Geometry: final body of the model. Coordinates: model frame, mm. A direction names the side the tool comes from. Round coordinates to 2 decimals unless told otherwise and drop trailing zeros. Write each loop counter-clockwise with the first axis right and the second up, starting at its lowest first coordinate (ties: lowest second). Pieces come first, ordered by that corner, then holes.
Autodesk Inventor part; units mm, degrees
ref_plane "YZ Plane" through (0, 0, 0) normal (1, 0, 0) x (0, 1, 0)
ref_plane "XZ Plane" through (0, 0, 0) normal (0, 1, 0) x (-1, 0, 0)
ref_plane "XY Plane" through (0, 0, 0) normal (0, 0, 1) x (1, 0, 0)
sketch "Эскиз1" plane through (0, 0, 0) normal (0, 1, 0) x (-1, 0, 0)
  arc A0 (-11.2808, -5.3845) -> (-11.2808, 5.3845) centre (0, 0) ccw
  arc A1 (-6.7685, -3.2307) -> (-6.7685, 3.2307) centre (0, 0) ccw
  line L0 (-6.7685, -3.2307) -> (-11.2808, -5.3845)
  line L1 (-6.7685, 3.2307) -> (-11.2808, 5.3845)
  dimension "d0" = 25
  dimension "d1" = 15
extrude "Выдавливание1" add sketch "Эскиз1" along normal blind 8
sketch "Эскиз2" plane through (0, 8, 0) normal (0, 1, 0) x (1, 0, 0)
  line L0 (5.4983, 5.1008) -> (9.1638, 8.5014)
  arc A0 (11.2808, 5.3845) -> (11.2808, -5.3845) centre (0, 0) ccw
  arc A1 (11.2808, 5.3845) -> (11.2808, -5.3845) centre (0, 0) ccw
  line L1 (11.2808, -5.3845) -> (6.7685, -3.2307)
  arc A2 (6.7685, 3.2307) -> (6.7685, -3.2307) centre (0, 0) ccw
  line L2 (6.7685, 3.2307) -> (11.2808, 5.3845)
  arc A3 (6.7685, 3.2307) -> (6.7685, -3.2307) centre (0, 0) ccw
  line L3 (5.4983, -5.1008) -> (9.1638, -8.5014)
  point P0 (11.2808, -5.3845)
extrude "Выдавливание2" add sketch "Эскиз2" along normal blind 2 contours L0 A0 L2 A2 | A2 L1 A0 L3
sketch "Эскиз3" plane through (0, 8, 0) normal (0, 1, 0) x (1, 0, 0)
  arc A0 (2.2493, 8.197) -> (-2.2493, 8.197) centre (0, 0) ccw
  arc A1 (3.1548, 11.0588) -> (-3.1548, 11.0588) centre (0, 0) ccw
  line L0 (3.4451, 8.7967) -> (3.8116, 9.7325)
  arc A2 (9.1638, 8.5014) -> (9.1638, -8.5014) centre (0, 0) ccw
  arc A3 (5.4983, 5.1008) -> (5.4983, -5.1008) centre (0, 0) ccw
  line L1 (-3.4451, 8.7967) -> (-3.8116, 9.7325)
  arc A4 (3.8116, 9.7325) -> (3.1548, 11.0588) centre (2.8804, 10.0972) ccw
  arc A5 (2.2493, 8.197) -> (3.4451, 8.7967) centre (2.5139, 9.1613) ccw
  arc A6 (-3.1548, 11.0588) -> (-3.8116, 9.7325) centre (-2.8804, 10.0972) ccw
  arc A7 (-3.4451, 8.7967) -> (-2.2493, 8.197) centre (-2.5139, 9.1613) ccw
  arc A8 (-5.9741, 6.0464) -> (-5.8956, 7.3819) centre (-6.677, 6.7578) ccw
  line L2 (-5.8956, 7.3819) -> (-6.5228, 8.1672)
  arc A9 (-5.9741, 6.0464) -> (-8.2235, 2.1505) centre (0, 0) ccw
  arc A10 (-9.3407, 1.4148) -> (-8.2235, 2.1505) centre (-9.1909, 2.4035) ccw
  arc A11 (-6.5228, 8.1672) -> (-7.9998, 8.2615) centre (-7.3042, 7.5431) ccw
  line L3 (-9.3407, 1.4148) -> (-10.3344, 1.5653)
  arc A12 (-11.1546, 2.7973) -> (-10.3344, 1.5653) centre (-10.1846, 2.5541) ccw
  arc A13 (-7.9998, 8.2615) -> (-11.1546, 2.7973) centre (0, 0) ccw
  arc A14 (-8.2235, -2.1505) -> (-9.3407, -1.4148) centre (-9.1909, -2.4035) ccw
  line L4 (-9.3407, -1.4148) -> (-10.3344, -1.5653)
  arc A15 (-8.2235, -2.1505) -> (-5.9741, -6.0464) centre (0, 0) ccw
  arc A16 (-5.8956, -7.3819) -> (-5.9741, -6.0464) centre (-6.677, -6.7578) ccw
  arc A17 (-10.3344, -1.5653) -> (-11.1546, -2.7973) centre (-10.1846, -2.5541) ccw
  line L5 (-5.8956, -7.3819) -> (-6.5228, -8.1672)
  arc A18 (-7.9998, -8.2615) -> (-6.5228, -8.1672) centre (-7.3042, -7.5431) ccw
  arc A19 (-11.1546, -2.7973) -> (-7.9998, -8.2615) centre (0, 0) ccw
  arc A20 (-2.2493, -8.197) -> (-3.4451, -8.7967) centre (-2.5139, -9.1613) ccw
  line L6 (-3.4451, -8.7967) -> (-3.8116, -9.7325)
  arc A21 (-2.2493, -8.197) -> (2.2493, -8.197) centre (0, 0) ccw
  arc A22 (3.4451, -8.7967) -> (2.2493, -8.197) centre (2.5139, -9.1613) ccw
  arc A23 (-3.8116, -9.7325) -> (-3.1548, -11.0588) centre (-2.8804, -10.0972) ccw
  line L7 (3.4451, -8.7967) -> (3.8116, -9.7325)
  arc A24 (3.1548, -11.0588) -> (3.8116, -9.7325) centre (2.8804, -10.0972) ccw
  arc A25 (-3.1548, -11.0588) -> (3.1548, -11.0588) centre (0, 0) ccw
  point P0 (4.1936, 10.7081)
  point P1 (3.0996, 7.9147)
  point P2 (-4.1936, 10.7081)
  point P3 (-3.0996, 7.9147)
  point P4 (-5.3045, 6.6417)
  point P5 (-8.4041, 1.273)
  point P6 (-7.1767, 8.9859)
  point P7 (-11.3703, 1.7222)
  point P8 (-8.4041, -1.273)
  point P9 (-5.3045, -6.6417)
  point P10 (-11.3703, -1.7222)
  point P11 (-7.1767, -8.9859)
  point P12 (-3.0996, -7.9147)
  point P13 (3.0996, -7.9147)
  point P14 (-4.1936, -10.7081)
  point P15 (4.1936, -10.7081)
  dimension "d8" = 3
  dimension "d9" = 1
  dimension "d12" = 180
extrude "Выдавливание3" cut sketch "Эскиз3" against normal blind 1
properties part number "pawn"
1) Section D-D on z = 0. Output: boundary loops of the cut face in (x, y).
2) Section C-C on y = 9. Output: boundary loops of the cut face in (x, z), plus the area to 3 significant figures.
3) First-contact query: P1, Ø3, axis at x = -9.5, z = -5.5, coming from the +Y side; P2, Ø1, axis at x = 1.5, z = -9.5, coming from the +Y side; P3, Ø1, axis at x = -5, z = 8.5, coming from the -Y side; P4, Ø1.5, axis at x = -4, y = 2.5, coming from the -Z side. Flat tips, straight axial feed; report the tip coordinate or a pass-through.
4) Draft query along X for faces 3 (the flat face through (8.99, 4.93, -4.29)), 4 (the flat face through (7.31, 8.99, 6.78)), 5 (the cylindrical face through (3.77, 7.51, 10.55)). Return one class per face: pulls with the +X half, pulls with the -X half, needs draft (parallel to the pull), parting line crosses it, or undercut.
5) Reachability of faces 1 (the cylindrical face through (-11.01, 7.51, 1.99)), 2 (the flat face through (8, 10, -6)) from +Z, -Z, +X, -X, +Y, -Y: full face, straight path, thin tool, end or side. Return the list, or none.
6) Section A-A on x = 0. Output: boundary loops of the cut face in (y, z), plus the area to 3 significant figures.
7) Line query: probe 1 along Z at (x, y) = (0, 3.25); probe 2 along Z at (x, y) = (-4, 1.5); probe 3 along X at (y, z) = (2.5, 0). Output: solid intervals per line, ascending.
8) Section B-B on z = -4.25. Output: boundary loops of the cut face in (x, y), plus the area to 3 significant figures.
Filled in:
1. outline: (-12.5, 0) - (-7.5, 0) - (-7.5, 8) - (-12.5, 8) - close
2. outline: (5.5, -5.1) - (9.16, -8.5) arc R12.5 ccw to (11.28, -5.38) - (6.77, -3.23) arc R7.5 cw to start; (5.5, 5.1) arc R7.5 cw to (6.77, 3.23) - (11.28, 5.38) arc R12.5 ccw to (9.16, 8.5) - close
2. area: 30.3 mm2
3. P1: stops at y = 8
3. P2: stops at y = 7
3. P3: stops at y = 0
3. P4: stops at z = -12.07
4. face 3: pulls with the +X half
4. face 4: pulls with the -X half
4. face 5: undercut
5. face 1: +Y
5. face 2: +Z, -Z, +X, -X, +Y
6. outline: (0, -12.5) - (8, -12.5) - (8, -11.5) - (7, -11.5) - (7, -8.5) - (8, -8.5) - (8, -7.5) - (0, -7.5) - close; (0, 7.5) - (8, 7.5) - (8, 8.5) - (7, 8.5) - (7, 11.5) - (8, 11.5) - (8, 12.5) - (0, 12.5) - close
6. area: 74.0 mm2
7. probe 1: z = -12.5 to -7.5, 7.5 to 12.5
7. probe 2: z = -11.84 to -6.34, 6.34 to 11.84
7. probe 3: x = -12.5 to -7.5
8. outline: (-11.76, 0) - (-6.18, 0) - (-6.18, 8) - (-7.36, 8) - (-7.36, 7) - (-10.69, 7) - (-10.69, 8) - (-11.76, 8) - close; (6.18, 0) - (8.9, 0) - (8.9, 10) - (6.18, 10) - close
8. area: 68.5 mm2
